from build123d import *

# Parameters (mm, degrees)
F2_R     = 43
F2_R_2   = 41
F0_DEPTH = 120.65
F3_R     = 43.053
F1_DEPTH = 3.5


with BuildPart() as f0:
    # F2 (on Top) → F0 (new body)
    with BuildSketch(Plane.XY):
        Circle(F2_R)
        Circle(F2_R_2, mode=Mode.SUBTRACT)
    extrude(amount=F0_DEPTH)

    # F3 (on Top) → F1 (join)
    with BuildSketch(Plane.XY):
        Circle(F3_R)
    extrude(amount=-F1_DEPTH)


solid = f0.part
Input: part model. Units: mm. Frame: model coordinates. Give positions to 0.01 mm unless a question says otherwise; leave off trailing zeros. Loops run counter-clockwise (first coordinate to the right, second up) from the corner with the lowest first, then second, coordinate; pieces in that order, holes last. Notation, with made-up numbers: (-21, 53.25) -> (24, 53.25) arc R12 ccw to (24, 66.25) -> close; hole circle Ø3 at (82.5, -16.5). An arc over 180 degrees is marked (long way). Answer as a JSON object with one key per item and string values. Group by question number.
Item 1: Pin query (flat end, axial travel): P1, Ø1.5, axis at x = 19, y = -2, coming from the +Z side; P2, Ø10, axis at y = -8, z = 42, coming from the -X side; P3, Ø10, axis at y = 21.5, z = 67, coming from the +X side. Return the tip coordinate at first contact, or that it passes through.
Item 2: Cut plane B-B, the plane z = 50.5. Return the cut outline in (x, y), and give its area (3 significant figures).
Item 3: Cut plane A-A, the plane y = 0. Return the cut outline in (x, z), and give its area (3 significant figures).
Item 4: Pull-direction query (X, two-part tool) for faces 1 (the cylindrical face through (-9, -40, 59)), 2 (the flat face through (-1, 1, 0)), 3 (the flat face through (38, -16, 120.65)), 4 (the cylindrical face through (-5.598, 42.634, 59.48)); classes: released by +X, released by -X, zero draft, split by the parting line, or undercut.
Item 5: Line query: probe 1 along Y at (x, z) = (0, 62); probe 2 along Z at (x, y) = (5, -26); probe 3 along X at (y, z) = (-37, 74.5). Output: solid intervals per line, ascending.
Checks:
{
 "1": {"P1": "stops at z = 0", "P2": "stops at x = -42.9", "P3": "stops at x = 39.71"},
 "2": {"outline": "circle Ø86 at (0, 0); hole circle Ø82 at (0, 0)", "area": "528 mm²"},
 "3": {"outline": "(-43.05, -3.5) -> (43.05, -3.5) -> (43.05, 0) -> (43, 0) -> (43, 120.65) -> (41, 120.65) -> (41, 0) -> (-41, 0) -> (-41, 120.65) -> (-43, 120.65) -> (-43, 0) -> (-43.05, 0) -> close", "area": "784 mm²"},
 "4": {"face 1": "undercut", "face 2": "undercut", "face 3": "zero draft", "face 4": "split by the parting line"},
 "5": {"probe 1": "y = -43 to -41, 41 to 43", "probe 2": "z = -3.5 to 0", "probe 3": "x = -21.91 to -17.66, 17.66 to 21.91"}
}
